Could you check a few things on this model? Use its own coordinates, in mm. A direction names the side the tool comes from. Coordinates: 2 decimals unless noted, no trailing zeros. Write each loop counter-clockwise with the first axis right and the second up, starting at its lowest first coordinate (ties: lowest second). Pieces come first, ordered by that corner, then holes. Notation, with made-up numbers: M 40.5,68.5 L 70.5,68.5 A16 ccw 70.5,73.5 Z; hole C 26.5,54 d10. An arc over 180 degrees is marked long. Write item = value, one per line.
```python
from build123d import *

# Parameters (mm, degrees)
F0_W     = 101.6
F0_H     = 101.6
F1_DEPTH = 101.6
F3_DEPTH = 121.666
F4_W     = 25.4
F4_H     = 76.2
F5_DEPTH = 50.8
F7_DEPTH = 99.568


with BuildPart() as f1:
    # F0 (on Front) → F1 (new body)
    with BuildSketch(Plane.XZ):
        with Locations((-50.8, -50.8)):
            Rectangle(F0_W, F0_H)
    extrude(amount=F1_DEPTH)

    # F2 (on face) → F3 (cut)
    with BuildSketch(Plane.YZ):
        Polygon((-50.8, -25.4), (-50.8, 0), (-101.6, 0), (-101.6, -76.2), (-25.4, -76.2), (-25.4, -25.4), align=None)
    extrude(amount=-F3_DEPTH, mode=Mode.SUBTRACT)

    # F4 (on face) → F5 (join)
    with BuildSketch(Plane.XY.offset(-76.2)):
        with Locations((-50.8, -63.5)):
            Rectangle(F4_W, F4_H)
    extrude(amount=F5_DEPTH)

    # F6 (on face) → F7 (cut)
    with BuildSketch(Plane.YZ.offset(-38.1)):
        Polygon((-101.6, -76.2), (-50.8, -25.4), (-92.064753, -25.4), (-101.6, -25.4), align=None)
    extrude(amount=-F7_DEPTH, mode=Mode.SUBTRACT)


solid = f1.part
```
Item 1: For faces 4 (the face through (0, -16, -63)), 5 (the face through (-19, -25.4, -51)), 6 (the face through (-52, -25, 0)), 7 (the face through (-82, -38, -25.4)), 8 (the face through (-50, -50.8, -13)), which set-ups out of +Z, -Z, +X, -X, +Y, -Y let a thin tool reach every point of the face, with its end or its side?
Numbers:
face_4 = +Z, -Z, +X, +Y, -Y
face_5 = +X, -Y
face_6 = +Z, +X, -X, +Y, -Y
face_7 = -X, -Y
face_8 = +Z, +X, -X, -Y
Item 2: Imagine slicing it at C-C (z = -13). Write out the boundary of the cut face in (x, y).
Numbers:
outline = M -101.6,-50.8 L 0,-50.8 L 0,0 L -101.6,0 Z
Item 3: If I drill on line 1 along Z through (x, y) = (-90, -49); line 2 along Y through (x, z) = (-5, -64.5); line 3 along X through (y, z) = (-36, -39.5), over which ranges is the centre line in solid material (lowest first)?
Numbers:
line_1 = -101.6 to -76.2, -25.4 to 0
line_2 = -25.4 to 0
line_3 = -63.5 to -38.1
Item 4: Imagine slicing it at D-D (y = -28.5). Write out the boundary of the cut face in (x, z).
Numbers:
outline = M -101.6,-101.6 L 0,-101.6 L 0,-76.2 L -38.1,-76.2 L -38.1,-25.4 L 0,-25.4 L 0,0 L -101.6,0 L -101.6,-25.4 L -63.5,-25.4 L -63.5,-76.2 L -101.6,-76.2 Z
Item 5: I'm going to push flat-ended pins straight in: P1, Ø1, axis at y = -62, z = -46, coming from the -X side; P2, Ø8, axis at x = -55, z = -53, coming from the -Y side; P3, Ø12.5, axis at x = -30, z = -18.5, coming from the -Y side. Where does each tip first touch, or does it pass through?
Numbers:
P1 = -63.5
P2 = -82.4
P3 = -50.8
Item 6: If we mould it in two halves opening along Z, with no side actions, what happens to faces 1 (the face through (-52, 0, -50)), 2 (the face through (-82, -25.4, -51)), 3 (the face through (-52, -50, -101.6))? For each: pulls with the +Z half, pulls with the -Z half, needs draft (parallel to the pull), parting line crosses it, or undercut.
Numbers:
face_1 = needs draft
face_2 = undercut
face_3 = pulls with the -Z half
Item 7: Imagine slicing it at B-B (y = -90.5). Write out the boundary of the cut face in (x, z).
Numbers:
outline = M -101.6,-101.6 L 0,-101.6 L 0,-76.2 L -38.1,-76.2 L -38.1,-65.1 L -63.5,-65.1 L -63.5,-76.2 L -101.6,-76.2 Z
Item 8: Imagine slicing it at A-A (x = -28). Write out the boundary of the cut face in (y, z).
Numbers:
outline = M -101.6,-101.6 L 0,-101.6 L 0,0 L -50.8,0 L -50.8,-25.4 L -25.4,-25.4 L -25.4,-76.2 L -101.6,-76.2 Z
